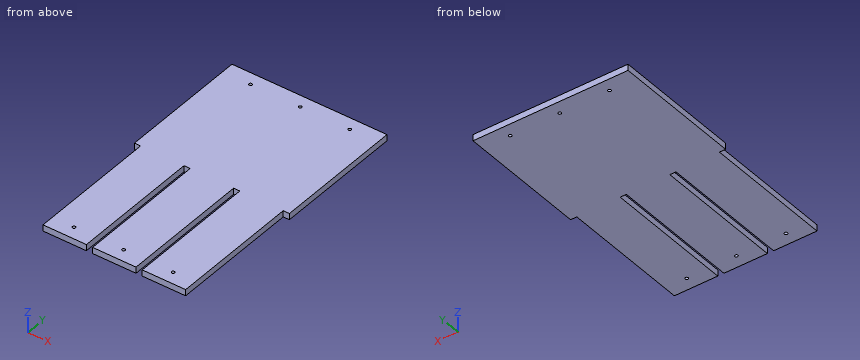
```python
from build123d import *

# Parameters (mm, degrees)
F0_W     = 22.225
F0_H     = 120.65
F1_DEPTH = 6.35
F3_D     = 3.175


# Not quite as in the source:
# - a feature names something its author has since deleted; it is built from what else it names


with BuildPart() as f1:
    # F0 (on Top) → F1 (new body)
    with BuildSketch(Plane.XY):
        Polygon((73.025, 133.35), (-73.025, 133.35), (-73.025, 120.65), (-50.8, 120.65), (0, 120.65), (50.8, 120.65), (73.025, 120.65), align=None)
        Polygon((-50.8, -120.65), (-73.025, -120.65), (-73.025, -133.35), (-28.575, -133.35), (-28.575, -120.65), align=None)
        Polygon((73.025, -133.35), (73.025, -120.65), (50.8, -120.65), (28.575, -120.65), (28.575, -133.35), align=None)
        with Locations((-61.9125, 60.325)):
            Rectangle(F0_W, F0_H)
        with Locations((-61.9125, -60.325)):
            Rectangle(F0_W, F0_H)
        with Locations((61.9125, 60.325)):
            Rectangle(F0_W, F0_H)
        with Locations((61.9125, -60.325)):
            Rectangle(F0_W, F0_H)
        Polygon((50.8, 0), (50.8, 120.65), (0, 120.65), (0, 0), (22.225, 0), (28.575, 0), align=None)
        Polygon((22.225, -120.65), (0, -120.65), (-22.225, -120.65), (-22.225, -133.35), (22.225, -133.35), align=None)
        Polygon((0, 120.65), (-50.8, 120.65), (-50.8, 0), (-28.575, 0), (-22.225, 0), (0, 0), align=None)
        with Locations((-39.6875, -60.325)):
            Rectangle(F0_W, F0_H)
        with Locations((-11.1125, -60.325)):
            Rectangle(F0_W, F0_H)
        with Locations((11.1125, -60.325)):
            Rectangle(F0_W, F0_H)
        with Locations((39.6875, -60.325)):
            Rectangle(F0_W, F0_H)
        Polygon((79.375, 133.35), (73.025, 133.35), (73.025, 120.65), (73.025, 0), (79.375, 0), align=None)
        Polygon((-73.025, 120.65), (-73.025, 133.35), (-79.375, 133.35), (-79.375, 0), (-73.025, 0), align=None)
    extrude(amount=F1_DEPTH)

    # F3 (through all)
    with Locations(Plane.XY.offset(6.35)):
        with Locations((-50.8, 120.65), (0, 120.65), (50.8, 120.65), (50.8, -120.65), (0, -120.65), (-50.8, -120.65)):
            Hole(F3_D / 2)


solid = f1.part
```
Read the model definition and answer for the solid it produces. Units are mm, in the model's axes. Give positions to 0.01 mm unless a question says otherwise; leave off trailing zeros. Loops run counter-clockwise (first coordinate to the right, second up) from the corner with the lowest first, then second, coordinate; pieces in that order, holes last.
Item 1: The part is cut by section B-B (z = 4.75). Give the number of separate pieces and of enclosed holes in the cut face, and give its area (3 significant figures).
Item 2: Each of these flat-tipped pins is pushed along its axis until it touches: pin 1 Ø1.9 at (y, z) = (-35, 4.5) entering from +X (3 decimals); pin 2 Ø3 at (x, z) = (77, 3) entering from -Y; pin 3 Ø2 at (y, z) = (-100.5, 1) entering from -X (3 decimals). Where does it stop, or does it pass through?
Item 3: Find the intervals of material crossed by line 1 along X through (y, z) = (-32.5, 1.75) (3 decimals); line 2 along Y through (x, z) = (50.8, 2); line 3 along X through (y, z) = (120.65, 3.25) (1 decimal), in increasing order.
Item 4: The part is cut by section A-A (y = -27). Write down the section's boundary in (x, z) (3 decimals), and give its area (3 significant figures).
Taken from the geometry:
1. separate pieces: 1
1. enclosed holes: 6
1. area: 38,900 mm2
2. pin 1: stops at x = 73.025
2. pin 2: stops at y = 0
2. pin 3: stops at x = -73.025
3. line 1: x = -73.025 to -28.575, -22.225 to 22.225, 28.575 to 73.025
3. line 2: y = -133.35 to -122.24, -119.06 to 119.06, 122.24 to 133.35
3. line 3: x = -79.4 to -52.4, -49.2 to -1.6, 1.6 to 49.2, 52.4 to 79.4
4. outline: (-73.025, 0) - (-28.575, 0) - (-28.575, 6.35) - (-73.025, 6.35) - close; (-22.225, 0) - (22.225, 0) - (22.225, 6.35) - (-22.225, 6.35) - close; (28.575, 0) - (73.025, 0) - (73.025, 6.35) - (28.575, 6.35) - close
4. area: 847 mm2
